Geometry: see drawing. Coordinates: mm, zero at the bounding-box minimum. A direction names the side the tool comes from. Coordinates: 2 decimals unless noted, no trailing zeros. Write each loop counter-clockwise with the first axis right and the second up, starting at its lowest first coordinate (ties: lowest second). Pieces come first, ordered by that corner, then holes. Notation, with made-up numbers: M 74.25,-25 L 92.25,-25 A22 ccw 92.25,5 Z; hole C 0.5,28 d5. An arc over 180 degrees is marked long. One line per item, written item: value. Start each with the question number.
Item 1: Pin query (flat end, axial travel): P1, Ø6, axis at x = 13.5, y = 14.5, coming from the +Z side; P2, Ø5, axis at x = 8.4, y = 8.4, coming from the -Z side. Return the tip coordinate at first contact, or that it passes through.
Item 2: Set-up query: the marked faces 4, 5 and 6. Return all of +Z, -Z, +X, -X, +Y, -Y with unobstructed straight access to the full face (end or side cutting, diameter ignored); none if empty.
Item 3: Cut plane A-A, the plane x = 8.4. Output: boundary loops of the cut face in (y, z).
Item 4: Cut plane B-B, the plane z = 3.85. Output: boundary loops of the cut face in (x, y), then the cut area to 3 significant figures.
Item 5: Ray query, L1, parallel to Y at x = 8.4, z = 4.1; L2, parallel to Y at x = 8.4, z = 4.75. Return the intervals inside material, ascending. Write a range as from..to.
Item 6: Cut plane C-C, the plane y = 14.75. Output: boundary loops of the cut face in (x, z).
Item 7: Mould query, pull axis Y, two halves, no side actions, for the marked faces 1, 2 and 3. Classes: released by +Y, released by -Y, zero draft, split by the parting line, or undercut.
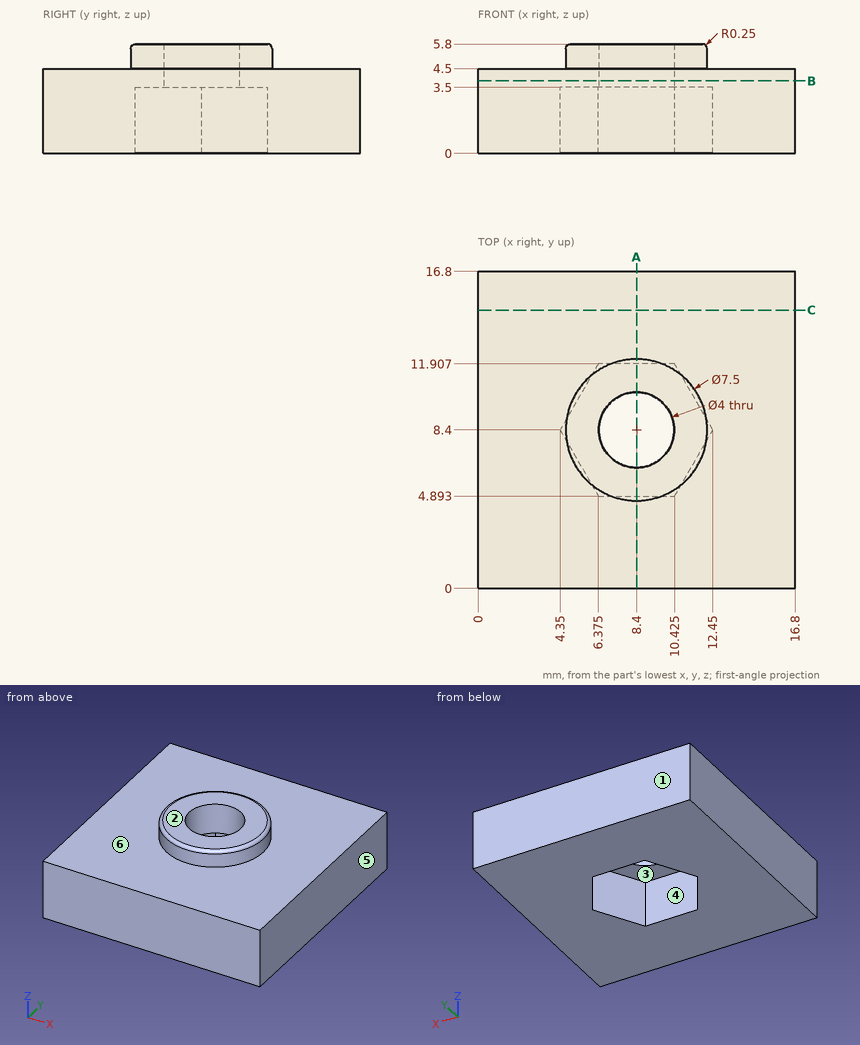
From the geometry:
1. P1: stops at z = 4.5
1. P2: stops at z = 3.5
2. face 4: -Z
2. face 5: +Z, -Z, +X, +Y, -Y
2. face 6: +Z
3. outline: M 0,0 L 4.89,0 L 4.89,3.5 L 6.4,3.5 L 6.4,5.8 L 4.9,5.8 A0.25 ccw 4.65,5.55 L 4.65,4.5 L 0,4.5 Z; M 10.4,3.5 L 11.91,3.5 L 11.91,0 L 16.8,0 L 16.8,4.5 L 12.15,4.5 L 12.15,5.55 A0.25 ccw 11.9,5.8 L 10.4,5.8 Z
4. outline: M 0,0 L 16.8,0 L 16.8,16.8 L 0,16.8 Z; hole C 8.4,8.4 d4
4. area: 270 mm²
5. L1: y = 0..6.4, 10.4..16.8
5. L2: y = 4.65..6.4, 10.4..12.15
6. outline: M 0,0 L 16.8,0 L 16.8,4.5 L 0,4.5 Z
7. face 1: released by +Y
7. face 2: zero draft
7. face 3: undercut
